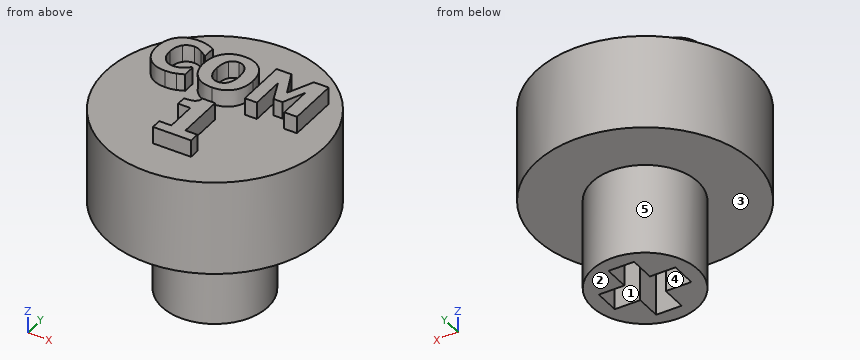
Autodesk Inventor part; units mm, degrees
ref_plane "YZ Plane" through (0, 0, 0) normal (1, 0, 0) x (0, 1, 0)
ref_plane "XZ Plane" through (0, 0, 0) normal (0, 1, 0) x (-1, 0, 0)
ref_plane "XY Plane" through (0, 0, 0) normal (0, 0, 1) x (1, 0, 0)
sketch "Sketch1" plane through (0, 0, 0) normal (0, 0, 1) x (1, 0, 0)
  circle A0 centre (0, 0) radius 6.22 construction
  circle A1 centre (0, 0) radius 2.8
  line L0 (-0.675, 0.675) -> (-0.675, 2.025)
  line L1 (-0.675, 2.025) -> (0.675, 2.025)
  line L2 (0.675, 2.025) -> (0.675, 0.675)
  line L3 (0.675, 0.675) -> (2.025, 0.675)
  line L4 (2.025, 0.675) -> (2.025, -0.675)
  line L5 (2.025, -0.675) -> (0.675, -0.675)
  line L6 (0.675, -0.675) -> (0.675, -2.025)
  line L7 (0.675, -2.025) -> (-0.675, -2.025)
  line L8 (-0.675, -2.025) -> (-0.675, -0.675)
  line L9 (-0.675, -0.675) -> (-2.025, -0.675)
  line L10 (-2.025, -0.675) -> (-2.025, 0.675)
  line L11 (-2.025, 0.675) -> (-0.675, 0.675)
  circle A2 centre (0, 0) radius 5.75
  point P0 (-6.07, -6.1)
  dimension "d0" = 12.44
  dimension "d1" = 0.47
extrude "Extrusion1" add sketch "Sketch1" along normal blind 5 contours A1 | L0 L1 L2 L3 L4 L5 L6 L7 L8 L9 L10 L11 | A2
extrude "Extrusion2" add sketch "Sketch1" against normal blind 4.8 contours A1
sketch "Sketch2" plane through (0, 0, 5) normal (0, 0, 1) x (1, 0, 0)
  point P0 (0, 0)
sketch "Sketch3" plane through (0, 0, 5) normal (0, 0, 1) x (1, 0, 0)
  line L0 (-4.2566, 3.1068) -> (4.2414, 3.1068) construction
  line L1 (4.2414, 3.1068) -> (4.2414, 0.2437) construction
  line L2 (4.2414, 0.2437) -> (-4.2566, 0.2437) construction
  line L3 (-4.2566, 0.2437) -> (-4.2566, 3.1068) construction
  line L4 (-1.3588, -0.6738) -> (1.3131, -0.6738) construction
  line L5 (1.3131, -0.6738) -> (1.3131, -3.7312) construction
  line L6 (1.3131, -3.7312) -> (-1.3588, -3.7312) construction
  line L7 (-1.3588, -3.7312) -> (-1.3588, -0.6738) construction
  spline S0 degree 2 poles (-2.8125, 0.2974) (-3.4208, 0.2974) (-4.1341, 1.0326) (-4.1341, 1.6977) knots 0 0 0 1 2 2 2
  spline S1 degree 2 poles (-4.1341, 1.6977) (-4.1341, 2.3388) (-3.4186, 3.1024) (-2.8103, 3.1024) knots 0 0 0 1 2 2 2
  spline S2 degree 2 poles (-2.8103, 3.1024) (-2.6506, 3.1024) (-2.3924, 3.0652) (-2.2743, 3.0346) knots 0 0 0 1 2 2 2
  spline S3 degree 2 poles (-2.2743, 3.0346) (-2.1824, 3.0062) (-1.9658, 2.9121) (-1.898, 2.8771) knots 0 0 0 1 2 2 2
  line L8 (-1.898, 2.8771) -> (-1.898, 2.2338)
  line L9 (-1.898, 2.2338) -> (-1.9658, 2.2338)
  spline S4 degree 2 poles (-1.9658, 2.2338) (-2.0161, 2.2775) (-2.1649, 2.4001) (-2.259, 2.457) knots 0 0 0 1 2 2 2
  spline S5 degree 2 poles (-2.259, 2.457) (-2.3531, 2.516) (-2.5784, 2.597) (-2.7031, 2.597) knots 0 0 0 1 2 2 2
  spline S6 degree 2 poles (-2.7031, 2.597) (-2.8497, 2.597) (-3.0926, 2.5051) (-3.2042, 2.3891) knots 0 0 0 1 2 2 2
  spline S7 degree 2 poles (-3.2042, 2.3891) (-3.3048, 2.2863) (-3.4339, 1.934) (-3.4339, 1.6955) knots 0 0 0 1 2 2 2
  spline S8 degree 2 poles (-3.4339, 1.6955) (-3.4339, 1.4439) (-3.3005, 1.1004) (-3.1911, 0.9954) knots 0 0 0 1 2 2 2
  spline S9 degree 2 poles (-3.1911, 0.9954) (-3.086, 0.8925) (-2.8279, 0.8028) (-2.6988, 0.8028) knots 0 0 0 1 2 2 2
  spline S10 degree 2 poles (-2.6988, 0.8028) (-2.5653, 0.8028) (-2.3224, 0.8925) (-2.2393, 0.9472) knots 0 0 0 1 2 2 2
  spline S11 degree 2 poles (-2.2393, 0.9472) (-2.1474, 1.0019) (-2.0095, 1.1179) (-1.9592, 1.1639) knots 0 0 0 1 2 2 2
  line L10 (-1.9592, 1.1639) -> (-1.898, 1.1639)
  line L11 (-1.898, 1.1639) -> (-1.898, 0.5293)
  spline S12 degree 2 poles (-1.898, 0.5293) (-1.9723, 0.4943) (-2.1671, 0.4068) (-2.2721, 0.3762) knots 0 0 0 1 2 2 2
  spline S13 degree 2 poles (-2.2721, 0.3762) (-2.399, 0.3368) (-2.62, 0.2974) (-2.8125, 0.2974) knots 0 0 0 1 2 2 2
  spline S14 degree 2 poles (0.9596, 1.6999) (0.9596, 1.0435) (0.2594, 0.293) (-0.3488, 0.293) knots 0 0 0 1 2 2 2
  spline S15 degree 2 poles (-0.3488, 0.293) (-0.9593, 0.293) (-1.6551, 1.0523) (-1.6551, 1.6999) knots 0 0 0 1 2 2 2
  spline S16 degree 2 poles (-1.6551, 1.6999) (-1.6551, 2.3498) (-0.9593, 3.1068) (-0.3488, 3.1068) knots 0 0 0 1 2 2 2
  spline S17 degree 2 poles (-0.3488, 3.1068) (0.2594, 3.1068) (0.9596, 2.3541) (0.9596, 1.6999) knots 0 0 0 1 2 2 2
  spline S18 degree 2 poles (0.2594, 1.6999) (0.2594, 1.9428) (0.161, 2.2819) (0.0756, 2.3891) knots 0 0 0 1 2 2 2
  spline S19 degree 2 poles (0.0756, 2.3891) (-0.0097, 2.5007) (-0.2285, 2.597) (-0.3467, 2.597) knots 0 0 0 1 2 2 2
  spline S20 degree 2 poles (-0.3467, 2.597) (-0.4714, 2.597) (-0.6749, 2.5073) (-0.7689, 2.3935) knots 0 0 0 1 2 2 2
  spline S21 degree 2 poles (-0.7689, 2.3935) (-0.8521, 2.2885) (-0.9549, 1.9406) (-0.9549, 1.6999) knots 0 0 0 1 2 2 2
  spline S22 degree 2 poles (-0.9549, 1.6999) (-0.9549, 1.4505) (-0.8565, 1.1223) (-0.7711, 1.0107) knots 0 0 0 1 2 2 2
  spline S23 degree 2 poles (-0.7711, 1.0107) (-0.6858, 0.8991) (-0.4648, 0.8028) (-0.3467, 0.8028) knots 0 0 0 1 2 2 2
  spline S24 degree 2 poles (-0.3467, 0.8028) (-0.2263, 0.8028) (-0.0031, 0.9057) (0.0778, 1.0151) knots 0 0 0 1 2 2 2
  spline S25 degree 2 poles (0.0778, 1.0151) (0.1653, 1.1332) (0.2594, 1.4461) (0.2594, 1.6999) knots 0 0 0 1 2 2 2
  line L12 (4.1191, 0.3499) -> (3.4452, 0.3499)
  line L13 (3.4452, 0.3499) -> (3.4452, 2.1397)
  line L14 (3.4452, 2.1397) -> (2.955, 0.9844)
  line L15 (2.955, 0.9844) -> (2.4912, 0.9844)
  line L16 (2.4912, 0.9844) -> (2.0011, 2.1397)
  line L17 (2.0011, 2.1397) -> (2.0011, 0.3499)
  line L18 (2.0011, 0.3499) -> (1.3622, 0.3499)
  line L19 (1.3622, 0.3499) -> (1.3622, 3.0499)
  line L20 (1.3622, 3.0499) -> (2.1433, 3.0499)
  line L21 (2.1433, 3.0499) -> (2.7428, 1.7174)
  line L22 (2.7428, 1.7174) -> (3.3379, 3.0499)
  line L23 (3.3379, 3.0499) -> (4.1191, 3.0499)
  line L24 (4.1191, 3.0499) -> (4.1191, 0.3499)
  line L25 (1.056, -3.7312) -> (-0.9584, -3.7312)
  line L26 (-0.9584, -3.7312) -> (-0.9584, -3.1998)
  line L27 (-0.9584, -3.1998) -> (-0.3157, -3.1998)
  line L28 (-0.3157, -3.1998) -> (-0.3157, -1.5858)
  line L29 (-0.3157, -1.5858) -> (-0.9584, -1.5858)
  line L30 (-0.9584, -1.5858) -> (-0.9584, -1.089)
  spline S26 degree 2 poles (-0.9584, -1.089) (-0.8175, -1.089) (-0.5382, -1.052) (-0.4541, -1.0124) knots 0 0 0 1 2 2 2
  spline S27 degree 2 poles (-0.4541, -1.0124) (-0.3578, -0.963) (-0.249, -0.7974) (-0.2391, -0.6738) knots 0 0 0 1 2 2 2
  line L31 (-0.2391, -0.6738) -> (0.4282, -0.6738)
  line L32 (0.4282, -0.6738) -> (0.4282, -3.1998)
  line L33 (0.4282, -3.1998) -> (1.056, -3.1998)
  line L34 (1.056, -3.1998) -> (1.056, -3.7312)
  point P0 (0, 0)
  point P1 (-0.0076, 0.2437)
  point P2 (-0.0228, -3.7312)
extrude "Extrusion3" add sketch "Sketch3" along normal blind 0.9
properties part number "IPC Com 1 key"
Geometry: final body of the model. Coordinates: model frame, mm. Face numbers are marked on the shaded views. A direction names the side the tool comes from. Round coordinates to 2 decimals unless told otherwise and drop trailing zeros. Order: outer loops, then holes, each group sorted by start corner. A loop starts at its lowest first (then second) coordinate and runs counter-clockwise, first axis right, second up. Notation, with made-up numbers: (17.5, 21.5) -> (43.5, 21.5) arc R10 ccw to (43.5, 37.5) -> close; hole circle Ø5 at (53.25, -1.75). An arc over 180 degrees is marked (long way). Write each question's results on one line, items separated by ' | '.
Q1. Section query A-A (z = -1). Output: boundary loops of the cut face in (x, y) (3 decimals), and give its area (3 significant figures).
Response values:
outline: circle Ø5.6 at (0, 0); hole (-2.025, -0.675) -> (-0.675, -0.675) -> (-0.675, -2.025) -> (0.675, -2.025) -> (0.675, -0.675) -> (2.025, -0.675) -> (2.025, 0.675) -> (0.675, 0.675) -> (0.675, 2.025) -> (-0.675, 2.025) -> (-0.675, 0.675) -> (-2.025, 0.675) -> close | area: 15.5 mm²
Q2. Section query C-C (x = 3.75). Output: boundary loops of the cut face in (y, z), and give its area (3 significant figures).
Response values:
outline: (-4.36, 0) -> (4.36, 0) -> (4.36, 5) -> (3.05, 5) -> (3.05, 5.9) -> (0.35, 5.9) -> (0.35, 5) -> (-4.36, 5) -> close | area: 46.0 mm²
Q3. Pull-direction query (Y, two-part tool) for the marked faces 3, 4 and 5; classes: released by +Y, released by -Y, zero draft, split by the parting line, or undercut.
Response values:
face 3: zero draft | face 4: undercut | face 5: split by the parting line
Q4. Ray query, line 1 along Z through (x, y) = (0, -3); line 2 along X through (y, z) = (-3.5, 5.5); line 3 along Z through (x, y) = (2, -4). Return the intervals inside material, ascending.
Response values:
line 1: 0 to 5.9 | line 2: -0.96 to 1.06 | line 3: 0 to 5
Q5. Access query for the marked faces 1 and 2. Directions: +Z, -Z, +X, -X, +Y, -Y. A direction counts if a zero-diameter tool reaches every point of the face in a straight line with its end or side. Return the directions, or none.
Response values:
face 1: -Z | face 2: -Z, +X, -X, +Y, -Y
Q6. Section query B-B (y = 0). Output: boundary loops of the cut face in (x, z) (3 decimals).
Response values:
outline: (-5.75, 0) -> (-2.8, 0) -> (-2.8, -4.8) -> (-2.025, -4.8) -> (-2.025, 0) -> (2.025, 0) -> (2.025, -4.8) -> (2.8, -4.8) -> (2.8, 0) -> (5.75, 0) -> (5.75, 5) -> (-5.75, 5) -> close
Q7. Section query D-D (z = 1.25). Output: boundary loops of the cut face in (x, y), and give its area (3 significant figures).
Response values:
outline: circle Ø11.5 at (0, 0) | area: 104 mm²
Q8. Pin query (flat end, axial travel): pin 1 Ø6 at (y, z) = (-3.5, -0.5) entering from -X; pin 2 Ø0.7 at (y, z) = (1.5, -2) entering from -X; pin 3 Ø4 at (x, z) = (4, 1.5) entering from +Y. Return the tip coordinate at first contact, or that it passes through.
Response values:
pin 1: x = -5.72 | pin 2: x = -2.55 | pin 3: y = 5.39
